Check sheet for the modelled part. Datum: model origin and axes. Units: mm. A direction names the side the tool comes from. Round coordinates to 2 decimals unless told otherwise and drop trailing zeros. Order: outer loops, then holes, each group sorted by start corner. A loop starts at its lowest first (then second) coordinate and runs counter-clockwise, first axis right, second up. Notation, with made-up numbers: M 78,3 L 118,3 A17 cw 118,21 Z; hole C 47,32 d5. An arc over 180 degrees is marked long. One line per item, written item: value. Start each with the question number.
(1) Thickness scan on L1, parallel to Z at x = -2.5, y = 26.6; L2, parallel to Y at x = 0, z = 17. Record the ranges inside material, lowest first.
(2) Cross-section at C-C, the plane x = -22.5. Enter the section's corners in (y, z), and give its area (3 significant figures).
(3) Cross-section at B-B, the plane z = 13.5. Enter the section's corners in (x, y).
(4) Depth check by flat-ended pin: pin 1 Ø4.5 at (x, z) = (-19, 10.5) entering from -Y; pin 2 Ø4.5 at (x, y) = (0, 0) entering from +Z; pin 3 Ø4 at (x, z) = (26.5, 13.5) entering from +Y; pin 4 Ø6 at (y, z) = (-17.5, 17.5) entering from -X. Enter the tip coordinate at first touch or a pass-through.
(5) Access from +Z, -Z, +X, -X, +Y, -Y to the whole of each face (thin tool, end or side, straight path). Record for faces 1 (the face through (27, 5, 10)), 2 (the face through (-13, 25, 12)), 3 (the face through (3, 4, 5)).
(6) Release check for a two-part mould opening along Z. For faces 4 (the face through (-3.71, 27.535, 11.897)), 5 (the face through (30, -13, 10)), 6 (the face through (27.535, -20.354, 10.676)), 7 (the face through (0, 7, 0)) record: released by +Z, released by -Z, zero draft, split by the parting line, or undercut.
(7) Cross-section at A-A, the plane z = 10. Enter the section's corners in (x, y).
from build123d import *

# Parameters (mm, degrees)
F0_W     = 35
F0_H     = 5
F0_W_2   = 5
F0_H_2   = 35
F1_DEPTH = 5
F2_W     = 35
F2_H     = 5
F2_W_2   = 5
F2_H_2   = 35
F3_DEPTH = 15
F4_R     = 2.5
F5_DEPTH = 5
F6_R     = 2.25
F7_DEPTH = 5
F8_R     = 2.25
F9_DEPTH = 5
F10_R    = 10


with BuildPart() as f1:
    # F0 (on Top) → F1 (new body)
    with BuildSketch(Plane.XY):
        Polygon((10.502526, -30), (25, -30), (25, 5), (5, 25), (-30, 25), (-30, 10.502526), (-19.747754, 0.250279), (0.251263, -19.748737), align=None)
        with Locations((-12.5, 27.5)):
            Rectangle(F0_W, F0_H)
        with Locations((27.5, -12.5)):
            Rectangle(F0_W_2, F0_H_2)
    extrude(amount=F1_DEPTH)

    # F2 (on face) → F3 (join)
    with BuildSketch(Plane.XY.offset(5)):
        with Locations((-12.5, 27.5)):
            Rectangle(F2_W, F2_H)
        with Locations((27.5, -12.5)):
            Rectangle(F2_W_2, F2_H_2)
    extrude(amount=F3_DEPTH)

    # F4 (on face) → F5 (cut, through all)
    with BuildSketch(Plane.XY.offset(5)):
        Circle(F4_R)
    extrude(amount=-F5_DEPTH, mode=Mode.SUBTRACT)

    # F6 (on face) → F7 (cut, through all)
    with BuildSketch(Plane.YZ.offset(30)):
        with Locations((-22.5, 10)):
            Circle(F6_R)
        with Locations((-2.5, 10)):
            Circle(F6_R)
    extrude(amount=-F7_DEPTH, mode=Mode.SUBTRACT)

    # F8 (on face) → F9 (cut, through all)
    with BuildSketch(Plane(origin=(0, 30, 0), x_dir=(-1, 0, 0), z_dir=(0, 1, 0))):
        with Locations((2.5, 10)):
            Circle(F8_R)
        with Locations((22.5, 10)):
            Circle(F8_R)
    extrude(amount=-F9_DEPTH, mode=Mode.SUBTRACT)

    # F10
    f10_edges = [f1.edges().sort_by_distance(p)[0] for p in [
        (-30, 10.502526, 2.5),
        (10.502526, -30, 2.5),
    ]]
    fillet(f10_edges, radius=F10_R)


solid = f1.part
Values found:
1. L1: 0 to 7.75, 12.25 to 20
1. L2: 25 to 30
2. outline: M 3,0 L 30,0 L 30,7.75 L 25,7.75 L 25,5 L 3,5 Z; M 25,12.25 L 30,12.25 L 30,20 L 25,20 Z
2. area: 187 mm^2
3. outline: M -30,25 L 5,25 L 5,30 L -30,30 Z; M 25,-30 L 30,-30 L 30,5 L 25,5 Z
4. pin 1: y = 25
4. pin 2: through
4. pin 3: y = 5
4. pin 4: x = 25
5. face 1: +Z, -Z, +X, +Y
5. face 2: +Z, +X, -X, -Y
5. face 3: +Z, -X, -Y
6. face 4: undercut
6. face 5: zero draft
6. face 6: undercut
6. face 7: released by -Z
7. outline: M -30,25 L -24.75,25 L -24.75,30 L -30,30 Z; M -20.25,25 L -4.75,25 L -4.75,30 L -20.25,30 Z; M -0.25,25 L 5,25 L 5,30 L -0.25,30 Z; M 25,-30 L 30,-30 L 30,-24.75 L 25,-24.75 Z; M 25,-20.25 L 30,-20.25 L 30,-4.75 L 25,-4.75 Z; M 25,-0.25 L 30,-0.25 L 30,5 L 25,5 Z
